The model under review builds one solid part; all positions refer to its coordinate system, in mm. Coordinates: 2 decimals unless noted, no trailing zeros. Write each loop counter-clockwise with the first axis right and the second up, starting at its lowest first coordinate (ties: lowest second). Pieces come first, ordered by that corner, then holes. Notation, with made-up numbers: M 29.5,42.5 L 33.5,42.5 A10 cw 33.5,50.5 Z; hole C 77,13 d6. An arc over 180 degrees is marked long. Answer as a JSON object with one key per item and string values.
```python
from build123d import *

# Parameters (mm, degrees)
SKETCH1_R            = 217
SKETCH1_R_2          = 190
MAINRING_DEPTH       = 10
M6_CLEARANCE_HOLE1_D = 6.6
HOLEPATTERN_COUNT    = 8
CUT_EXTRUDE1_DEPTH   = 11
CIRPATTERN1_COUNT    = 8


with BuildPart() as part:
    # Sketch1 → MainRing (new body)
    with BuildSketch(Plane(origin=(0, 0, 0), x_dir=(1, 0, 0), z_dir=(0, 1, 0))):
        Circle(SKETCH1_R)
        Circle(SKETCH1_R_2, mode=Mode.SUBTRACT)
    extrude(amount=MAINRING_DEPTH)

    # M6 Clearance Hole1 (through all)
    with Locations(Plane(origin=(0, 0, 0), x_dir=(-1, 0, 0), z_dir=(0, -1, 0))):
        with Locations((0, -204.5)):
            m6_clearance_hole1 = Hole(M6_CLEARANCE_HOLE1_D / 2)

    # HolePattern: M6 Clearance Hole1 ×8 about axis
    holepattern_axis = Axis((0, 0, 0), (0, 1, 0))
    for i in range(1, HOLEPATTERN_COUNT):
        add(m6_clearance_hole1.rotate(holepattern_axis, i * 360 / HOLEPATTERN_COUNT), mode=Mode.SUBTRACT)

    # Sketch5 → Cut-Extrude1 (cut, through all)
    with BuildSketch(Plane.XZ):
        with BuildLine():
            ThreePointArc((201.13360859, -5.168316504), (204.040552386, -15.742991514), (207.729432581, -5.415056739))
            ThreePointArc((207.729432581, -5.415056739), (207.782357396, -2.707758263), (207.8, 0))
            ThreePointArc((207.8, 0), (204.5, -3.3), (201.2, 0))
            ThreePointArc((201.2, 0), (201.183401463, -2.584371456), (201.13360859, -5.168316504))
        make_face()
    cut_extrude1 = extrude(amount=-CUT_EXTRUDE1_DEPTH, mode=Mode.SUBTRACT)

    # CirPattern1: Cut-Extrude1 ×8 about axis
    cirpattern1_axis = Axis((0, 0, 0), (0, 1, 0))
    for i in range(1, CIRPATTERN1_COUNT):
        add(cut_extrude1.rotate(cirpattern1_axis, i * 360 / CIRPATTERN1_COUNT), mode=Mode.SUBTRACT)


solid = part.part
```
(1) For pin 1 Ø2 at (x, y) = (-117, 6.5) entering from +Z; pin 2 Ø4 at (y, z) = (7.5, -115) entering from -X; pin 3 Ø1 at (x, y) = (170.5, 8.5) entering from -Z; pin 4 Ø7 at (x, z) = (151.5, 137.36) entering from +Y, all flat-tipped, find the tip position at first contact; note any pin that passes through.
Results list:
{"pin 1": "z = 183.39", "pin 2": "x = -185.26", "pin 3": "z = -134.87", "pin 4": "through"}
(2) Add section B-B on x = -99. Give the boundary of the cut face in (y, z), and give its area (3 significant figures).
Results list:
{"outline": "M 0,-193.1 L 10,-193.1 L 10,-162.17 L 0,-162.17 Z; M 0,162.17 L 10,162.17 L 10,193.1 L 0,193.1 Z", "area": "619 mm²"}
(3) Draft analysis for pull direction Z (two halves, no side actions). For faces 1 (the face through (-1, 0, 192)), 2 (the face through (-133.01, 4.93, 155.26)), 3 (the face through (206.98, 4.93, -65.18)), state which applies: released by +Z, released by -Z, zero draft, split by the parting line, or undercut.
Results list:
{"face 1": "zero draft", "face 2": "undercut", "face 3": "split by the parting line"}
(4) Wall thickness on line 1 along Z through (x, y) = (156, 2.25); line 2 along X through (y, z) = (8.75, 140); line 3 along X through (y, z) = (8.5, -150): over which ranges is each line inside the solid? List them lowest first. Write a range as from..to.
Results list:
{"line 1": "-150.84..-108.46, 108.46..133.78, 140.94..150.84", "line 2": "-165.8..-128.45, 128.45..144.5, 156.61..165.8", "line 3": "-156.81..-116.62, 116.62..131.81, 143.81..156.81"}
(5) Add section A-A on z = -83. Give the boundary of the cut face in (x, y).
Results list:
{"outline": "M -200.5,0 L -170.91,0 L -170.91,10 L -200.5,10 Z; M 170.91,0 L 200.5,0 L 200.5,10 L 170.91,10 Z"}
(6) Add section C-C on y = 5.25. Count the separate pieces of the cut face and the enclosed holes in it, and give its area (3 significant figures).
Results list:
{"separate pieces": "1", "enclosed holes": "9", "area": "33,300 mm²"}
